Could you check a few things on this model? Use its own coordinates, in mm. A direction names the side the tool comes from. Give positions to 0.01 mm unless a question says otherwise; leave off trailing zeros. Loops run counter-clockwise (first coordinate to the right, second up) from the corner with the lowest first, then second, coordinate; pieces in that order, holes last. Notation, with made-up numbers: (49.5, 13.25) -> (107.5, 13.25) arc R17 ccw to (107.5, 19.25) -> close; hole circle Ø11 at (73.5, 41.5). An arc over 180 degrees is marked (long way). Put each result on its own line as item: value.
```python
from build123d import *

# Parameters (mm, degrees)
SKETCH1_R           = 6
SKETCH1_R_2         = 3
BOSS_EXTRUDE1_DEPTH = 1.4
BOSS_EXTRUDE2_START = -1.4
SKETCH3_R           = 6
SKETCH3_R_2         = 3.1
BOSS_EXTRUDE2_DEPTH = 1.4
SKETCH5_R           = 5.7
SKETCH5_R_2         = 3.3
BOSS_EXTRUDE4_DEPTH = 0.5
CIRPATTERN2_COUNT   = 9
CIRPATTERN2_2_COUNT = 9
CHAMFER1_SIZE       = 0.1


with BuildPart() as part:
    # Sketch1 → Boss-Extrude1 (new body)
    with BuildSketch(Plane(origin=(0, 0, 0), x_dir=(1, 0, 0), z_dir=(0, 1, 0))):
        with Locations(Location((0, 0, 0), (0, 0, 270))):
            Circle(SKETCH1_R)
        with Locations(Location((0, 0, 0), (0, 0, 270))):
            Circle(SKETCH1_R_2, mode=Mode.SUBTRACT)
    extrude(amount=BOSS_EXTRUDE1_DEPTH)


with BuildPart() as body_2:
    # Sketch3 → Boss-Extrude2 (new body)
    with BuildSketch(Plane(origin=(0, 4.5, 0), x_dir=(1, 0, 0), z_dir=(0, 1, 0)).offset(BOSS_EXTRUDE2_START)):
        with Locations(Location((0, 0, 0), (0, 0, 270))):
            Circle(SKETCH3_R)
        with Locations(Location((0, 0, 0), (0, 0, 270))):
            Circle(SKETCH3_R_2, mode=Mode.SUBTRACT)
    extrude(amount=BOSS_EXTRUDE2_DEPTH)


with BuildPart() as body_3:
    # Sketch5 → Boss-Extrude4 (new, symmetric)
    with BuildSketch(Plane(origin=(0, 2.25, 0), x_dir=(1, 0, 0), z_dir=(0, 1, 0))):
        with Locations(Location((0, 0, 0), (0, 0, 270))):
            Circle(SKETCH5_R)
        with Locations(Location((0, 0, 0), (0, 0, 270))):
            Circle(SKETCH5_R_2, mode=Mode.SUBTRACT)
    extrude(amount=BOSS_EXTRUDE4_DEPTH, both=True)


with BuildPart() as cut_revolve1_tool:
    # Sketch2 → Cut-Revolve1 (revolve)
    with BuildSketch(Plane(origin=(0, 2.25, 0), x_dir=(1, 0, 0), z_dir=(0, 1, 0))):
        with BuildLine():
            Line((-4.5, 1), (-4.5, -1))
            ThreePointArc((-4.5, -1), (-5.5, 0), (-4.5, 1))
        make_face()
    cut_revolve1 = revolve(axis=Axis((-4.5, 2.25, -1), (0, 0, 1)))


with BuildPart() as part_1:
    add(part.part)

    # Cut-Revolve1: cut by cut_revolve1_tool
    add(cut_revolve1_tool.part, mode=Mode.SUBTRACT)

    # Sketch2_3 → Revolve1 (revolve)
    with BuildSketch(Plane(origin=(0, 2.25, 0), x_dir=(1, 0, 0), z_dir=(0, 1, 0))):
        with BuildLine():
            Line((-4.5, 1), (-4.5, -1))
            ThreePointArc((-4.5, -1), (-5.5, 0), (-4.5, 1))
        make_face()
    revolve1 = revolve(axis=Axis((-4.5, 2.25, -1), (0, 0, 1)))


with BuildPart() as body_2_1:
    add(body_2.part)

    # Cut-Revolve1: cut by cut_revolve1_tool
    add(cut_revolve1_tool.part, mode=Mode.SUBTRACT)


with BuildPart() as body_3_1:
    add(body_3.part)

    # Cut-Revolve1: cut by cut_revolve1_tool
    add(cut_revolve1_tool.part, mode=Mode.SUBTRACT)


with BuildPart() as cirpattern2_tool:
    # CirPattern2: Cut-Revolve1 ×9 about axis
    cirpattern2_axis = Axis((0, 0, 0), (0, 1, 0))
    for i in range(1, CIRPATTERN2_COUNT):
        add(cut_revolve1.rotate(cirpattern2_axis, i * 360 / CIRPATTERN2_COUNT))


with BuildPart() as part_2:
    add(part_1.part)

    # CirPattern2: cut by cirpattern2_tool
    add(cirpattern2_tool.part, mode=Mode.SUBTRACT)



with BuildPart() as body_2_2:
    add(body_2_1.part)

    # CirPattern2: cut by cirpattern2_tool
    add(cirpattern2_tool.part, mode=Mode.SUBTRACT)


with BuildPart() as body_3_2:
    add(body_3_1.part)

    # CirPattern2: cut by cirpattern2_tool
    add(cirpattern2_tool.part, mode=Mode.SUBTRACT)


with BuildPart() as part_3:
    add(part_2.part)

    add(body_2_2.part)  # CirPattern2 2 merges body 2

    add(body_3_2.part)  # CirPattern2 2 merges body 3
    # CirPattern2 2: Revolve1 ×9 about axis
    cirpattern2_2_axis = Axis((0, 0, 0), (0, 1, 0))
    for i in range(1, CIRPATTERN2_2_COUNT):
        add(revolve1.rotate(cirpattern2_2_axis, i * 360 / CIRPATTERN2_2_COUNT))

    # Chamfer1
    chamfer1_edges = [part_3.edges().sort_by_distance(p)[0] for p in [
        (0, 3.1, -6),
        (0, 3.1, -3.1),
        (0, 4.5, -6),
        (0, 1.4, -6),
        (0, 0, -6),
        (0, 1.4, -3),
    ]]
    chamfer(chamfer1_edges, length=CHAMFER1_SIZE)


solid = part_3.part
```
1. If we section it at C-C (y = 3.7): List the corners of the cut face in (x, z) for me.
Recorded:
outline: circle Ø12 at (0, 0); hole circle Ø6.2 at (0, 0)
2. I need wall thicknesses on line 1 (Y direction, x = 2.25, z = -2.75); line 2 (X direction, y = 2.35, z = 0); line 3 (Y direction, x = -3, z = 1.25). Which ranges of each line are inside material? Lowest first, please.
Recorded:
line 1: y = 0 to 1.4, 1.75 to 2.75, 3.1 to 4.5
line 2: x = -5.7 to -3.3, 3.3 to 5.7
line 3: y = 0 to 1.4, 3.1 to 4.5
3. If we section it at A-A (y = 2.95): Count the separate pieces of the cut face and the enclosed holes in it, then the cut area to 3 significant figures.
Recorded:
separate pieces: 9
enclosed holes: 0
area: 14.4 mm^2
4. For faces 1 (the face through (-2.5, 3.1, 2.5)), 2 (the face through (1.802, 3.792, 5.723)), 3 (the face through (0.931, 3.841, 2.957)), which set-ups out of +Z, -Z, +X, -X, +Y, -Y let a thin tool reach every point of the face, with its end or its side?
Recorded:
face 1: none
face 2: +Y, -Y
face 3: +Y
5. Thinking about a two-plate mould opening in Z: for faces 4 (the face through (1.802, 0.692, 5.723)), 5 (the face through (-2.008, 2.243, -2.619)), 6 (the face through (-3, 4.5, 3)), which applies, pulls with the +Z half, pulls with the -Z half, needs draft (parallel to the pull), parting line crosses it, or undercut?
Recorded:
face 4: parting line crosses it
face 5: undercut
face 6: needs draft
6. I'm going to push flat-ended pins straight in: pin 1 (5 mm diameter, centred on x = 0, z = 0, fed in from +Y); pin 2 (1 mm diameter, centred on y = 1, z = 1.5, fed in from -X); pin 3 (1.5 mm diameter, centred on y = 3.5, z = -3.5, fed in from -X); pin 4 (2 mm diameter, centred on x = 5, y = 0.5, fed in from +Z). Where does each tip first touch, or does it pass through?
Recorded:
pin 1: passes through
pin 2: stops at x = -5.92
pin 3: stops at x = -5.33
pin 4: stops at z = 4.47
